Autodesk Inventor part; units mm, degrees
ref_plane "YZ Plane" through (0, 0, 0) normal (1, 0, 0) x (0, 1, 0)
ref_plane "XZ Plane" through (0, 0, 0) normal (0, 1, 0) x (-1, 0, 0)
ref_plane "XY Plane" through (0, 0, 0) normal (0, 0, 1) x (1, 0, 0)
sketch "スケッチ1" plane through (0, 0, 0) normal (1, 0, 0) x (0, 1, 0)
  line L0 (35, -49) -> (-5, -49)
  line L1 (-5, -49) -> (-5, -100)
  line L2 (-5, -100) -> (35, -100)
  line L3 (35, -100) -> (35, -49)
  dimension "d1" = 40
  dimension "d2" = 51
extrude "押し出し1" add sketch "スケッチ1" along normal blind 3
sketch "スケッチ4" plane through (3, 0, 0) normal (1, 0, 0) x (0, 0, -1)
  line L0 (54, 30) -> (95, 30)
  line L1 (95, 30) -> (95, 0)
  line L2 (95, 0) -> (54, 0)
  line L3 (54, 0) -> (54, 30)
  line L4 (100, 35) -> (49, 35)
  line L5 (100, -5) -> (100, 35)
  point P0 (0, 0)
  dimension "d29" = 41
  dimension "d30" = 30
  dimension "d31" = 5
  dimension "d32" = 5
hole "穴2" at (3, 30, -54) at (3, 0, -54) at (3, 0, -95) at (3, 30, -95) direction (-1, 0, 0) diameter 3.2 end through all
sketch "スケッチ6" plane through (3, 0, 0) normal (1, 0, 0) x (0, 0, -1)
  line L0 (49, 35) -> (49, -5)
  line L1 (49, 15) -> (100, 15)
  line L2 (100, -5) -> (100, 35)
  circle A0 centre (74.5, 15) radius 13.5
  point P0 (0, 0)
  point P1 (88, 15)
  point P2 (81.25, 26.6913)
  point P3 (67.75, 26.6913)
  point P4 (61, 15)
  point P5 (67.75, 3.3087)
  point P6 (81.25, 3.3087)
  dimension "d53" = 27
  dimension "d56" = 360
hole "穴4" at (3, 15, -88) at (3, 26.6913, -81.25) at (3, 26.6913, -67.75) at (3, 15, -61) at (3, 3.3087, -67.75) at (3, 3.3087, -81.25) direction (-1, 0, 0) diameter 3.2 end through all
properties part number "link5_plate2" material "アルミニウム 6061"
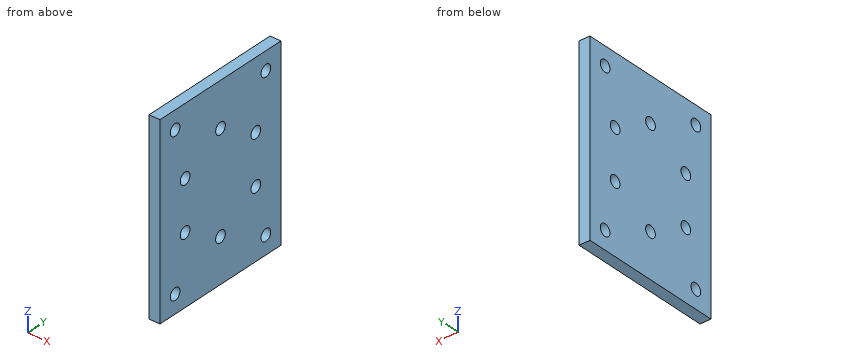
Geometry: final body of the model. Coordinates: model frame, mm. Coordinates: 2 decimals unless noted, no trailing zeros. Loops run counter-clockwise (first coordinate to the right, second up) from the corner with the lowest first, then second, coordinate; pieces in that order, holes last. Notation, with made-up numbers: M 14,86.25 L 21,86.25 A23 cw 21,105.25 Z; hole C 66.5,-19 d8. An arc over 180 degrees is marked long. Put each result on its own line as item: value.
(1) Cut plane C-C on x = 1.4. State how many separate pieces and enclosed holes the cut face has, then the cut area to 3 significant figures.
Answer sheet:
separate pieces: 1
enclosed holes: 10
area: 1,960 mm^2
(2) Material intervals for probe 1 along Y at (x, z) = (0.75, -95); probe 2 along Z at (x, y) = (2.3, 0); probe 3 along Y at (x, z) = (1.2, -67.75), sorted ascending.
Answer sheet:
probe 1: y = -5 to -1.6, 1.6 to 28.4, 31.6 to 35
probe 2: z = -100 to -96.6, -93.4 to -55.6, -52.4 to -49
probe 3: y = -5 to 1.71, 4.91 to 25.09, 28.29 to 35
(3) Cut plane B-B on z = -88. Return the cut outline in (x, y).
Answer sheet:
outline: M 0,-5 L 3,-5 L 3,13.4 L 0,13.4 Z; M 0,16.6 L 3,16.6 L 3,35 L 0,35 Z
(4) Cut plane D-D on y = 26. Return the cut outline in (x, z).
Answer sheet:
outline: M 0,-100 L 3,-100 L 3,-82.69 L 0,-82.69 Z; M 0,-79.81 L 3,-79.81 L 3,-69.19 L 0,-69.19 Z; M 0,-66.31 L 3,-66.31 L 3,-49 L 0,-49 Z
(5) First-contact query: pin 1 (3 mm diameter, centred on y = 15, z = -88, fed in from -X). Flat tip, straight axial feed; report the tip coordinate or a pass-through.
Answer sheet:
pin 1: passes through
(6) Cut plane A-A on z = -54. Return the cut outline in (x, y), then the cut area to 3 significant figures.
Answer sheet:
outline: M 0,-5 L 3,-5 L 3,-1.6 L 0,-1.6 Z; M 0,1.6 L 3,1.6 L 3,28.4 L 0,28.4 Z; M 0,31.6 L 3,31.6 L 3,35 L 0,35 Z
area: 101 mm^2
